Geometry check sheet. Reference: drawing and pictorial views, mm from the part's lowest x, y, z. Coordinates: 2 decimals unless noted, no trailing zeros. Write each loop counter-clockwise with the first axis right and the second up, starting at its lowest first coordinate (ties: lowest second). Pieces come first, ordered by that corner, then holes. Notation, with made-up numbers: (5, -29) -> (41, -29) arc R28 cw to (41, -11) -> close; hole circle Ø6 at (78.25, 5.5). An arc over 180 degrees is marked (long way). Use a Markdown table: item, result.
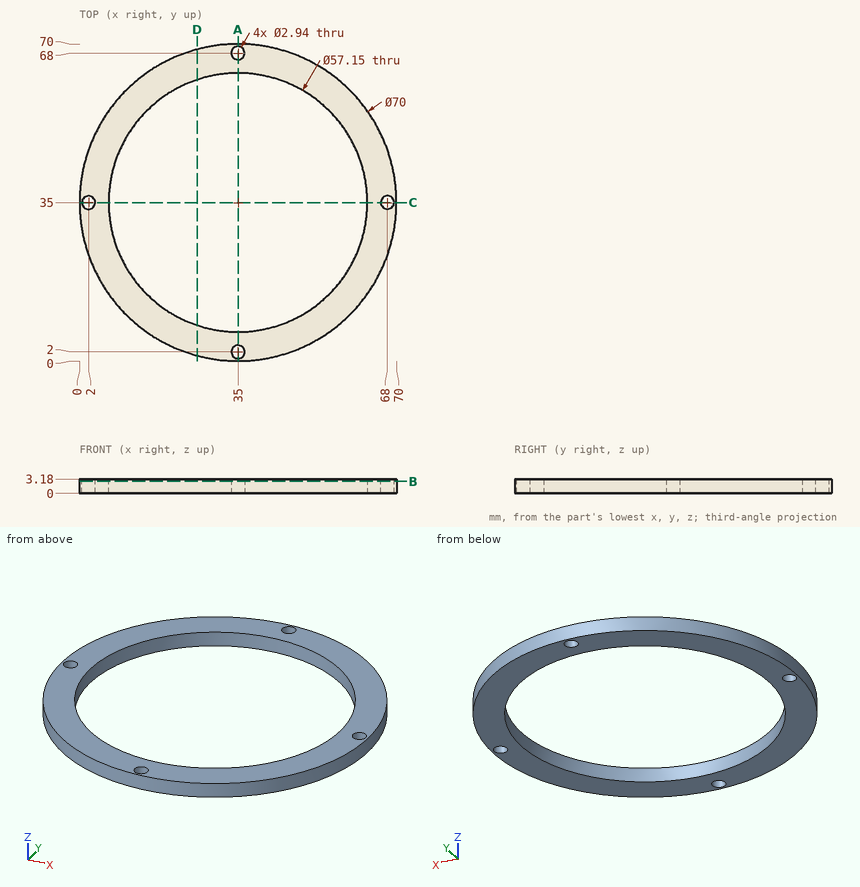
Item 1: Section check D-D on x = 26. Record the boundary of the cut face in (y, z).
Answer block:
| item | result |
|---|---|
| outline | (1.18, 0) -> (7.88, 0) -> (7.88, 3.18) -> (1.18, 3.18) -> close; (62.12, 0) -> (68.82, 0) -> (68.82, 3.18) -> (62.12, 3.18) -> close |
Item 2: Depth check by flat-ended pin: P1, Ø1.5, axis at x = 59, z = 3, coming from the +Y side; P2, Ø1.5, axis at x = 55.5, z = 1, coming from the -Y side. Enter the tip coordinate at first touch or a pass-through.
Answer block:
| item | result |
|---|---|
| P1 | stops at y = 61.16 |
| P2 | stops at y = 6.1 |
Item 3: Thickness scan on L1, parallel to Y at x = 35, z = 2.1 (3 decimals); L2, parallel to X at y = 49, z = 1.65; L3, parallel to Y at x = 44, z = 1.8. Record the ranges inside material, lowest first. Write a range as [from, to].
Answer block:
| item | result |
|---|---|
| L1 | y = [0, 0.53], [3.47, 6.425], [63.575, 66.53], [69.47, 70] |
| L2 | x = [2.92, 10.09], [59.91, 67.08] |
| L3 | y = [1.18, 7.88], [62.12, 68.82] |
Item 4: Section check A-A on x = 35. Record the boundary of the cut face in (y, z) (3 decimals).
Answer block:
| item | result |
|---|---|
| outline | (0, 0) -> (0.53, 0) -> (0.53, 3.18) -> (0, 3.18) -> close; (3.47, 0) -> (6.425, 0) -> (6.425, 3.18) -> (3.47, 3.18) -> close; (63.575, 0) -> (66.53, 0) -> (66.53, 3.18) -> (63.575, 3.18) -> close; (69.47, 0) -> (70, 0) -> (70, 3.18) -> (69.47, 3.18) -> close |
Item 5: Section check B-B on z = 2.65. Record the boundary of the cut face in (x, y) (3 decimals), then the cut area to 3 significant figures.
Answer block:
| item | result |
|---|---|
| outline | circle Ø70 at (35, 35); hole circle Ø2.94 at (2, 35); hole circle Ø57.15 at (35, 35); hole circle Ø2.94 at (35, 2); hole circle Ø2.94 at (35, 68); hole circle Ø2.94 at (68, 35) |
| area | 1,260 mm^2 |
